For this review, take the finished solid that the model builds, in its own axes (mm). A direction names the side the tool comes from. Round coordinates to 2 decimals unless told otherwise and drop trailing zeros. Loops run counter-clockwise (first coordinate to the right, second up) from the corner with the lowest first, then second, coordinate; pieces in that order, holes last.
1. To check wall thickness, follow line 1 along X through (y, z) = (-0.6, -2.1) (3 decimals); line 2 along Y through (x, z) = (6, 1.65); line 3 along Y through (x, z) = (5.5, 1.8). State the ranges of each line that lie inside material, in increasing order.
2. Clearance check with flat-ended pins moving along their axes: pin 1 Ø1.5 at (x, y) = (7.5, -0.5) entering from -Z; pin 2 Ø2 at (x, z) = (15.5, 1.5) entering from +Y. State where each tip first meets the part, or that it passes through.
3. Consider section C-C on x = 9.5. State the section outline as (y, z) points, then the cut area to 3 significant figures.
4. Tool access review of faces 1 (the cylindrical face through (3.219, 1.833, -0.76)), 2 (the flat face through (0, 0, 0)), 3 (the cylindrical face through (57.194, 1.833, -0.76)): name each direction out of +Z, -Z, +X, -X, +Y, -Y from which nothing blocks a thin tool from reaching the whole face with its end or side.
5. Consider section A-A on y = 0. State the section outline as (x, z) points (3 decimals).
Autodesk Inventor part; units mm, degrees
ref_plane "Start Plane" through (0, 0, 0) normal (1, 0, 0) x (0, 1, 0)
ref_plane "XZ Plane" through (0, 0, 0) normal (0, 1, 0) x (-1, 0, 0)
ref_plane "XY Plane" through (0, 0, 0) normal (0, 0, 1) x (1, 0, 0)
sketch "Main Sketch" plane through (0, 0, 0) normal (0, 0, 1) x (1, 0, 0)
  line L0 (0, 0) -> (60.325, 0)
  line L1 (0, 0) -> (0, 1.9844)
  line L2 (0, 1.9844) -> (6.35, 1.9844)
  line L3 (6.35, 1.9844) -> (6.35, 2.3813)
  line L4 (53.975, 2.3813) -> (53.975, 1.9844)
  line L5 (6.35, 2.3813) -> (53.975, 2.3813)
  line L6 (60.325, 1.9844) -> (60.325, 0)
  line L7 (53.975, 1.9844) -> (60.325, 1.9844)
  dimension "d3" = 3.9688
  dimension "d4" = 4.7625
  dimension "d5" = 3.9688
revolve "Revolution1" add sketch "Main Sketch" angle 360 about axis through (0, 0, 0) along (1, 0, 0)
equation "\"Length\" = 60.325"
properties part number "Shaft" material "Steel"
Resolved:
1. line 1: x = 6.35 to 53.975
1. line 2: y = -1.1 to 1.1
1. line 3: y = -0.84 to 0.84
2. pin 1: stops at z = -2.38
2. pin 2: stops at y = 2.33
3. outline: circle Ø4.76 at (0, 0)
3. area: 17.8 mm2
4. face 1: -X
4. face 2: +Z, -Z, -X, +Y, -Y
4. face 3: +X
5. outline: (0, -1.984) - (6.35, -1.984) - (6.35, -2.381) - (53.975, -2.381) - (53.975, -1.984) - (60.325, -1.984) - (60.325, 1.984) - (53.975, 1.984) - (53.975, 2.381) - (6.35, 2.381) - (6.35, 1.984) - (0, 1.984) - close
